from build123d import *

# Parameters (mm, degrees)
F0_W     = 57.15
F0_H     = 44.45
F1_DEPTH = 25.4
F3_DEPTH = 12.7
F5_DEPTH = 12.701
F7_DEPTH = 25.401


with BuildPart() as f1:
    # F0 (on Front) → F1 (new body)
    with BuildSketch(Plane.XZ):
        with Locations((28.575, 22.225)):
            Rectangle(F0_W, F0_H)
    extrude(amount=F1_DEPTH)

    # F2 (on face) → F3 (cut)
    with BuildSketch(Plane.XZ.offset(25.4)):
        Polygon((57.15, 44.45), (17.8654808551, 44.45), (43.8516363502, 0), (57.15, 0), align=None)
    extrude(amount=-F3_DEPTH, mode=Mode.SUBTRACT)

    # F4 (on face) → F5 (cut, through all)
    with BuildSketch(Plane.XZ.offset(12.7)):
        with BuildLine():
            ThreePointArc((33.3435072178, 17.9744302701), (37.1242051851, 21.7860579667), (38.5066656507, 26.9736379303))
            ThreePointArc((38.5066656507, 26.9736379303), (33.2700116001, 36.0154114789), (22.8213560552, 35.9728455904))
            Line((22.8213560552, 35.9728455904), (33.3435072178, 17.9744302701))
        make_face()
    extrude(amount=-F5_DEPTH, mode=Mode.SUBTRACT)

    # F6 (on face) → F7 (cut, through all)
    with BuildSketch(Plane.XZ.offset(25.4)):
        with BuildLine():
            Line((33.2805792258, 18.0820702495), (22.8900132849, 35.8554055997))
            ThreePointArc((22.8900132849, 35.8554055997), (18.8883674995, 21.5920715416), (33.2805792258, 18.0820702495))
        make_face()
    extrude(amount=-F7_DEPTH, mode=Mode.SUBTRACT)


solid = f1.part
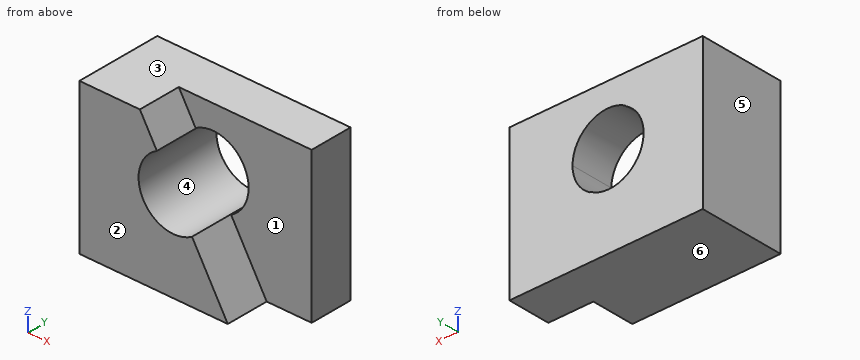
Read the model definition and answer for the solid it produces. Units are mm, in the model's axes. Face numbers are marked on the shaded views. A direction names the side the tool comes from. Round coordinates to 2 decimals unless told otherwise and drop trailing zeros. Write each loop counter-clockwise with the first axis right and the second up, starting at its lowest first coordinate (ties: lowest second). Pieces come first, ordered by that corner, then holes. Notation, with made-up numbers: (-39.5, -9) - (8.5, -9) arc R11 cw to (8.5, 9) - close; hole circle Ø10 at (80.5, -17). An arc over 180 degrees is marked (long way). One line per question, with ' | ' between items. Start each with the question number.
1. This flat-tipped pin is pushed along its axis until it touches: pin 1 (10 mm diameter, centred on x = 41.5, y = -21.5, fed in from -Z). Where does it stop, or does it pass through?
2. For a pull along Z with two mould halves and no side action, classify the marked faces 3, 4, 5 and 6 as +Z half, -Z half, draft (parallel to the pull), parting line (faces both ways), or undercut.
3. Section B-B (z = 20.5) is taken. Determine the outline of the cut face in (x, y), and give its area (3 significant figures).
4. For the marked faces 1 and 2, determine the directions among +Z, -Z, +X, -X, +Y, -Y from which every point of the face is accessible in a straight line to the end or side of a thin tool.
5. Find the intervals of material crossed by probe 1 along Y at (x, z) = (41.5, 41); probe 2 along X at (y, z) = (-8.5, 29); probe 3 along X at (y, z) = (-9, 33.5), in increasing order. Write a range as [from, to].
6. Section C-C (x = 32) is taken. Determine the outline of the cut face in (y, z).
7. Section A-A (y = -10) is taken. Determine the outline of the cut face in (x, z).
8. Section D-D (z = 12) is taken. Determine the outline of the cut face in (x, y), and give its area (3 significant figures).
Filled in:
1) pin 1: z = 0
2) face 3: +Z half | face 4: undercut | face 5: draft | face 6: -Z half
3) outline: (0, -25.4) - (19.62, -25.4) - (19.62, 0) - (0, 0) - close; (36.25, -12.7) - (57.15, -12.7) - (57.15, 0) - (36.25, 0) - close | area: 764 mm²
4) face 1: +Z, +X, -Y | face 2: +Z, -Z, +X, -X, -Y
5) probe 1: [-12.7, 0] | probe 2: [0, 17.72], [38.31, 57.15] | probe 3: [0, 19.97], [36.21, 57.15]
6) outline: (-25.4, 0) - (0, 0) - (0, 17.39) - (-25.4, 17.39) - close; (-12.7, 36.63) - (0, 36.63) - (0, 44.45) - (-12.7, 44.45) - close
7) outline: (0, 0) - (57.15, 0) - (57.15, 44.45) - (0, 44.45) - close; hole (22.82, 35.97) - (22.89, 35.86) arc R10.3 ccw (long way) to (33.28, 18.08) - (33.34, 17.97) arc R10.42 ccw to start
8) outline: (0, -25.4) - (36.84, -25.4) - (36.84, -12.7) - (57.15, -12.7) - (57.15, 0) - (0, 0) - close | area: 1,190 mm²
